Input: dimensioned drawing with shaded views. Units: mm. Origin: part minimum x, y, z. A direction names the side the tool comes from. Give positions to 0.01 mm unless a question says otherwise; leave off trailing zeros. Write each loop counter-clockwise with the first axis right and the second up, starting at its lowest first coordinate (ties: lowest second). Pieces come first, ordered by that corner, then holes.
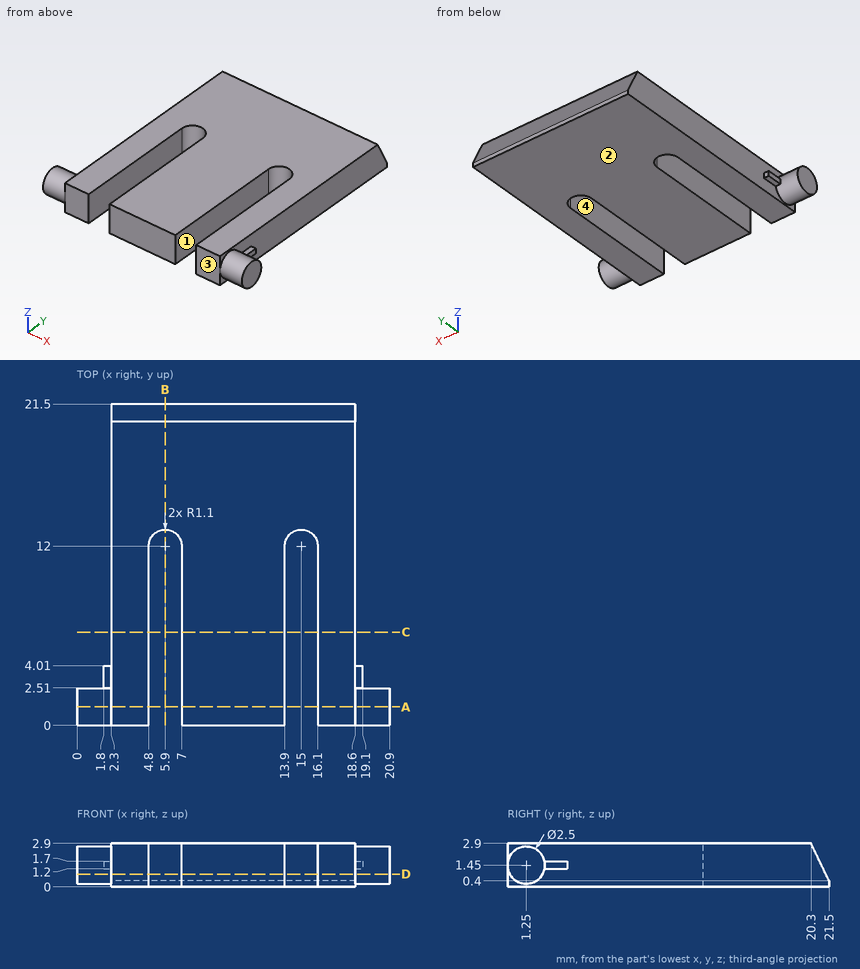
Item 1: Section B-B (x = 5.9). Return loops of the section in (y, z).
Item 2: Set-up query: the marked faces 1 and 2. Return all of +Z, -Z, +X, -X, +Y, -Y with unobstructed straight access to the full face (end or side cutting, diameter ignored); none if empty.
Item 3: Section A-A (y = 1.25). Return loops of the section in (x, z), and give its area (3 significant figures).
Item 4: Pin query (flat end, axial travel): pin 1 (0.9 mm diameter, centred on y = 8.5, z = 1, fed in from -X); pin 2 (0.6 mm diameter, centred on x = 19, z = 1.5, fed in from +Y); pin 3 (1.5 mm diameter, centred on x = 17, z = 2, fed in from +Y). Return the tip coordinate at first contact, or that it passes through.
Item 5: Section D-D (z = 0.85). Return loops of the section in (x, y).
Item 6: Mould query, pull axis X, two halves, no side actions, for the marked faces 3 and 4. Classes: +X half, -X half, draft (parallel to the pull), parting line (faces both ways), or undercut.
Item 7: Ray query, line 1 (X direction, y = 11, z = 2.3); line 2 (X direction, y = 18, z = 2.7); line 3 (Y direction, x = 5.5, z = 0.9). Return the intervals inside material, ascending.
Item 8: Section C-C (y = 6.25). Return loops of the section in (x, z), and give its area (3 significant figures).
Solved:
1. outline: (13.1, 0) - (21.5, 0) - (21.5, 0.4) - (20.3, 2.9) - (13.1, 2.9) - close
2. face 1: +Z, -Z, -Y
2. face 2: -Z, +X, -X, +Y, -Y
3. outline: (0, 0.2) - (2.3, 0.2) - (2.3, 0) - (4.8, 0) - (4.8, 2.9) - (2.3, 2.9) - (2.3, 2.7) - (0, 2.7) - close; (7, 0) - (13.9, 0) - (13.9, 2.9) - (7, 2.9) - close; (16.1, 0) - (18.6, 0) - (18.6, 0.2) - (20.9, 0.2) - (20.9, 2.7) - (18.6, 2.7) - (18.6, 2.9) - (16.1, 2.9) - close
3. area: 46.0 mm2
4. pin 1: stops at x = 2.3
4. pin 2: stops at y = 4.01
4. pin 3: stops at y = 21.09
5. outline: (0, 0.15) - (2.3, 0.15) - (2.3, 0) - (4.8, 0) - (4.8, 12) arc R1.1 cw to (7, 12) - (7, 0) - (13.9, 0) - (13.9, 12) arc R1.1 cw to (16.1, 12) - (16.1, 0) - (18.6, 0) - (18.6, 0.15) - (20.9, 0.15) - (20.9, 2.35) - (18.6, 2.35) - (18.6, 21.28) - (2.3, 21.28) - (2.3, 2.35) - (0, 2.35) - close
6. face 3: draft
6. face 4: undercut
7. line 1: x = 2.3 to 4.8, 7 to 13.9, 16.1 to 18.6
7. line 2: x = 2.3 to 18.6
7. line 3: y = 13.02 to 21.26
8. outline: (2.3, 0) - (4.8, 0) - (4.8, 2.9) - (2.3, 2.9) - close; (7, 0) - (13.9, 0) - (13.9, 2.9) - (7, 2.9) - close; (16.1, 0) - (18.6, 0) - (18.6, 2.9) - (16.1, 2.9) - close
8. area: 34.5 mm2
